Geometry: final body of the model. Coordinates: model frame, mm. A direction names the side the tool comes from. Give positions to 0.01 mm unless a question says otherwise; leave off trailing zeros. Write each loop counter-clockwise with the first axis right and the second up, starting at its lowest first coordinate (ties: lowest second). Pieces come first, ordered by that corner, then holes. Notation, with made-up numbers: (-28, 0.5) -> (-13, 0.5) arc R25 cw to (-13, 35.5) -> close; hole circle Ø5 at (58.5, -8). An arc over 180 degrees is marked (long way). Use CSV: the item, a comma, the result in double quotes. Start each with the question number.
1) Section C-C (z = -6.5). Output: boundary loops of the cut face in (x, y).
2) Contact query for flat-ended pins moving along their axis: P1, Ø2, axis at y = -3, z = 93, coming from the +X side; P2, Ø1.5, axis at x = 1, z = 146.5, coming from the -Y side; P3, Ø1.5, axis at x = 2, z = 144, coming from the +Y side. Output: stop coordinate, or through.
3) Section A-A (x = 0). Output: boundary loops of the cut face in (y, z) (1 decimal), plus the area to 3 significant figures.
4) Set-up query: faces 1 (the face through (-0.867, 3.905, 199.565)), 2 (the face through (0.867, 3.905, -10.846)), 3 (the face through (0, 0, -22)). Return all of +Z, -Z, +X, -X, +Y, -Y with unobstructed straight access to the full face (end or side cutting, diameter ignored); none if empty.
5) Section D-D (z = 108). Output: boundary loops of the cut face in (x, y) (1 decimal).
6) Material intervals for line 1 (X direction, y = -0.5, z = 77); line 2 (Z direction, x = 2.75, y = -3.75); line 3 (X direction, y = 0.75, z = -9), sorted ascending. Write a range as [from, to].
Autodesk Inventor part; units mm, degrees
ref_plane "YZ Plane" through (0, 0, 0) normal (1, 0, 0) x (0, 1, 0)
ref_plane "XZ Plane" through (0, 0, 0) normal (0, 1, 0) x (-1, 0, 0)
ref_plane "XY Plane" through (0, 0, 0) normal (0, 0, 1) x (1, 0, 0)
sketch "Sketch1" plane through (0, 0, 0) normal (0, 0, 1) x (1, 0, 0)
  circle A0 centre (0, 0) radius 4.7625
  dimension "d0" = 9.525
extrude "Extrusion1" add sketch "Sketch1" along normal blind 198
sketch "Sketch2" plane through (0, 0, 198) normal (0, 0, 1) x (1, 0, 0)
  circle A0 centre (0, 0) radius 4.7625
  circle A1 centre (0, 0) radius 4
  dimension "d4" = 8
extrude "Extrusion2" add sketch "Sketch2" along normal blind 3.175 contours A1
sketch "Sketch3" plane through (0, 0, 0) normal (0, 0, -1) x (-1, 0, 0)
  circle A0 centre (0, 0) radius 4.7625
  circle A1 centre (0, 0) radius 4
  dimension "d7" = 8
extrude "Extrusion3" add sketch "Sketch3" along normal blind 22 contours A1
thread "Thread1"
properties part number "S2_zrod"
Answers follow:
1,outline,"circle Ø8 at (0, 0)"
2,P1,"stops at x = 4.32"
2,P2,"stops at y = -4.76"
2,P3,"stops at y = 4.6"
3,outline,"(-4.8, 0) -> (-4, 0) -> (-4, -22) -> (4, -22) -> (4, 0) -> (4.8, 0) -> (4.8, 198) -> (4, 198) -> (4, 201.2) -> (-4, 201.2) -> (-4, 198) -> (-4.8, 198) -> close"
3,area,"2,090 mm^2"
4,face 1,"+Z"
4,face 2,"-Z"
4,face 3,"-Z, +X, -X, +Y, -Y"
5,outline,"circle Ø9.5 at (0, 0)"
6,line 1,"x = [-4.74, 4.74]"
6,line 2,"z = [0, 198]"
6,line 3,"x = [-3.93, 3.93]"
